Autodesk Inventor part; units mm, degrees
ref_plane "YZ Plane" through (0, 0, 0) normal (1, 0, 0) x (0, 1, 0)
ref_plane "XZ Plane" through (0, 0, 0) normal (0, 1, 0) x (-1, 0, 0)
ref_plane "XY Plane" through (0, 0, 0) normal (0, 0, 1) x (1, 0, 0)
sketch "Szkic1" plane through (0, 0, 0) normal (1, 0, 0) x (0, 1, 0)
  line L0 (-19.507, 0) -> (22.493, 0)
  line L1 (0, -18.291) -> (0, 5.509)
  line L2 (16.493, -14.891) -> (-13.507, -14.891)
  line L3 (-13.507, -14.891) -> (-13.507, 2.109)
  line L4 (16.493, -14.891) -> (16.493, 2.109)
  point P0 (0, 0)
  dimension "d1" = 30
  dimension "d2" = 17
  dimension "d3" = 17
contour flange "Kołnierz z profilu1" sketch "Szkic1" thickness 0.5 bend radius 0.5 width 184 along (1, 0, 0) mid plane no both sides no wall seen from (0, 16.493, -6.391) lies toward (0, -1, 0) curves L4 L2 L3
bend "Gięcie1"
corner "Narożnik1"
equation "\"d3\" = d2"
equation "\"d4\" = SzerokośćGięciaPodcięcia"
equation "\"d5\" = GłębokośćGięciaPodcięcia"
equation "\"d6\" = MinimalnaPozostałość"
equation "\"d7\" = PromieńGięcia"
equation "\"d9\" = PromieńGięcia"
equation "\"d11\" = RozmiarPodcięciaNarożnika"
equation "\"d12\" = Wielk_odstępu"
equation "\"d13\" = Rozmiar_promienia_Jacobiego"
equation "\"PromieńGięcia\" = Grubość"
equation "\"SzerokośćGięciaPodcięcia\" = Grubość"
equation "\"GłębokośćGięciaPodcięcia\" = 0.5 * Grubość"
equation "\"RozmiarPodcięciaNarożnika\" = 4 * Grubość"
equation "\"MinimalnaPozostałość\" = 2 * Grubość"
equation "\"PromieńPrzejścia\" = PromieńGięcia"
equation "\"Rozmiar_promienia_Jacobiego\" = PromieńGięcia"
equation "\"Wielk_odstępu\" = Grubość"
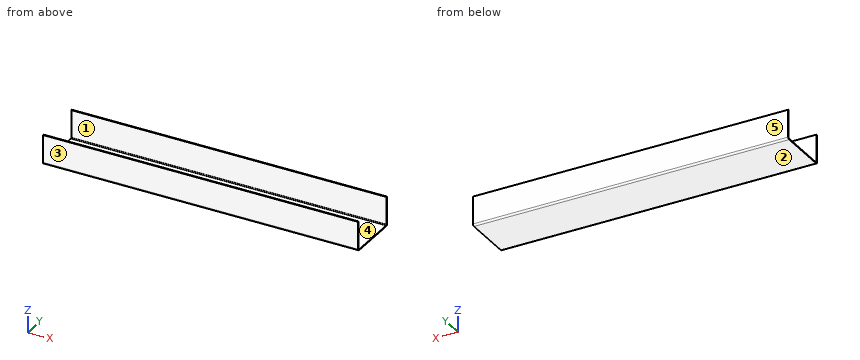
Part model, mm, in its own coordinate system. Face numbers are marked on the shaded views. A direction names the side the tool comes from. Round coordinates to 2 decimals unless told otherwise and drop trailing zeros. Order: outer loops, then holes, each group sorted by start corner. A loop starts at its lowest first (then second) coordinate and runs counter-clockwise, first axis right, second up. Notation, with made-up numbers: (7, 56.5) -> (37, 56.5) arc R11 cw to (37, 63.5) -> close; hole circle Ø2 at (38, 44.5). An arc over 180 degrees is marked (long way). Put each result on its own line as item: value.
Q1. Band-saw the part on A-A (z = -4). Give the cut face in (x, y).
From the geometry:
outline: (0, -13.51) -> (184, -13.51) -> (184, -13.01) -> (0, -13.01) -> close; (0, 15.99) -> (184, 15.99) -> (184, 16.49) -> (0, 16.49) -> close
Q2. Tool access for the marked faces 1 and 2: list every direction of +Z, -Z, +X, -X, +Y, -Y with a clear straight run to the whole face (end or side of a thin tool).
From the geometry:
face 1: +Z, +X, -X
face 2: -Z, +X, -X, +Y, -Y
Q3. Band-saw the part on B-B (x = 83.5). Give the cut face in (y, z), and give its area (3 significant figures).
From the geometry:
outline: (-13.51, -13.89) arc R1 ccw to (-12.51, -14.89) -> (15.49, -14.89) arc R1 ccw to (16.49, -13.89) -> (16.49, 2.11) -> (15.99, 2.11) -> (15.99, -13.89) arc R0.5 cw to (15.49, -14.39) -> (-12.51, -14.39) arc R0.5 cw to (-13.01, -13.89) -> (-13.01, 2.11) -> (-13.51, 2.11) -> close
area: 31.2 mm2
Q4. Band-saw the part on C-C (y = -2.5). Give the cut face in (x, z).
From the geometry:
outline: (0, -14.89) -> (184, -14.89) -> (184, -14.39) -> (0, -14.39) -> close
Q5. Pull direction Y, two halves, no side cores. Call the marked faces 3, 4 and 5: pulls with the +Y half, pulls with the -Y half, needs draft (parallel to the pull), parting line crosses it, or undercut.
From the geometry:
face 3: pulls with the -Y half
face 4: undercut
face 5: pulls with the +Y half
Q6. Pin check, flat tip, straight feed: pin 1 Ø3 at (x, y) = (23, -8) entering from +Z. Stop position of the tip, or through.
From the geometry:
pin 1: stops at z = -14.39
Q7. Wall check: line 1 (Y direction, x = 102, z = -14); line 2 (Z direction, x = 82.5, y = 9). Give the ranges that are in metal, low to high. Write a range as [from, to].
From the geometry:
line 1: y = [-13.5, -12.99], [15.98, 16.49]
line 2: z = [-14.89, -14.39]
